Check sheet for the drawn part. Datum: minimum x, y, z corner. Units: mm. Round coordinates to 2 decimals unless told otherwise and drop trailing zeros. Write each loop counter-clockwise with the first axis right and the second up, starting at its lowest first coordinate (ties: lowest second). Pieces come first, ordered by that corner, then holes. Notation, with made-up numbers: M 15,79 L 64,79 A18 ccw 64,99 Z; hole C 57,-12.75 d10. An arc over 180 degrees is marked long. One line per item, written item: value. Start each with the question number.
Item 1: Section check B-B, the plane z = 43.5. Record the cut outline in (x, y).
Item 2: Gauge pin test, flat ends, axial feed: pin 1 (8 mm diameter, centred on y = 21.5, z = 21.5, fed in from +X) (1 decimal); pin 2 (1.5 mm diameter, centred on x = 97, y = 16, fed in from -Z) (1 decimal); pin 3 (4 mm diameter, centred on y = 16.5, z = 13.5, fed in from +X). Record the tip position at first contact, or that the pin passes through.
Item 3: Section check D-D, the plane x = 102. Record the cut outline in (y, z), then the cut area to 3 significant figures.
Item 4: Draft check along X on the marked faces 1, 2, 3 and 4. Enter one of: +X half, -X half, draft (parallel to the pull), parting line (faces both ways), or undercut.
Item 5: Section check A-A, the plane x = 61. Record the cut outline in (y, z), then the cut area to 3 significant figures.
Item 6: Thickness scan on probe 1 along Z at (x, y) = (54.5, 42.5) (1 decimal); probe 2 along X at (y, z) = (3, 37) (1 decimal); probe 3 along X at (y, z) = (21, 74.5) (1 decimal). Record the ranges inside material, lowest first. Write a range as from..to.
Item 7: Section check C-C, the plane y = 11. Record the cut outline in (x, z) (1 decimal), then the cut area to 3 significant figures.
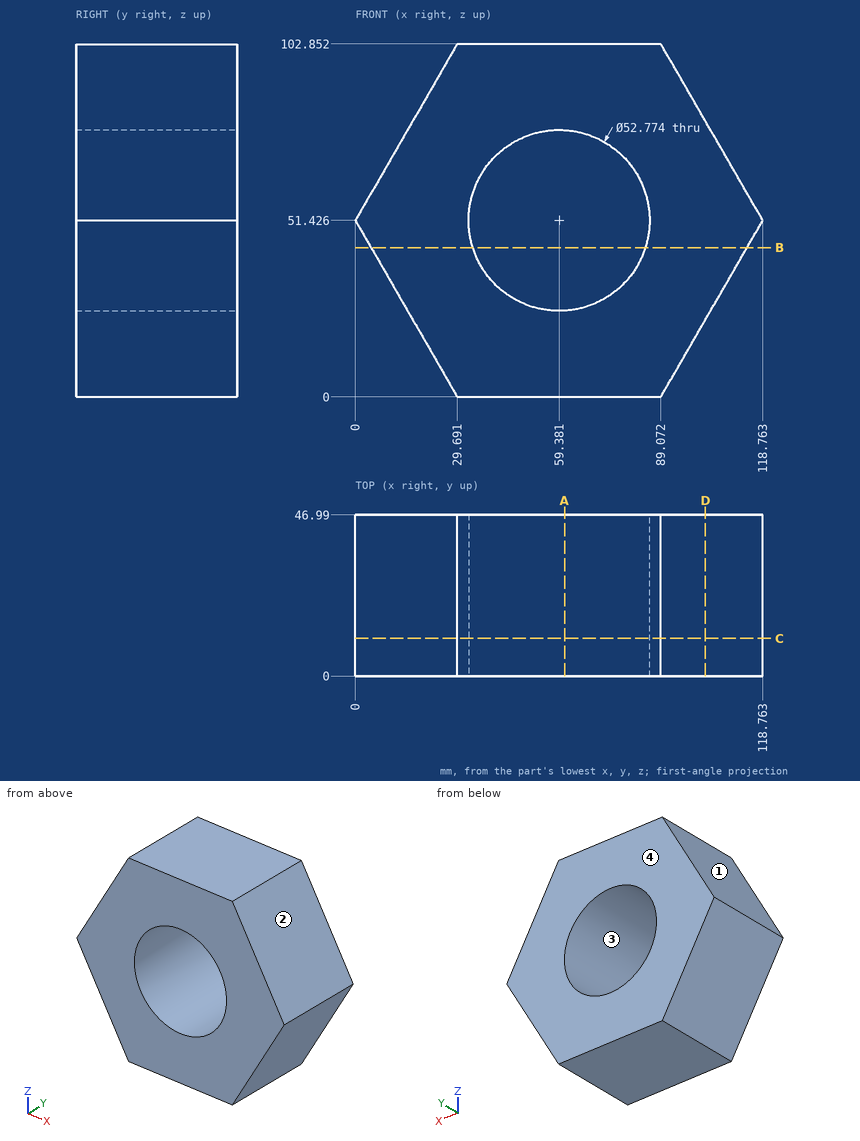
Response values:
1. outline: M 4.58,0 L 34.21,0 L 34.21,46.99 L 4.58,46.99 Z; M 84.55,0 L 114.19,0 L 114.19,46.99 L 84.55,46.99 Z
2. pin 1: stops at x = 103.8
2. pin 2: stops at z = 12.4
2. pin 3: stops at x = 98.02
3. outline: M 0,22.39 L 46.99,22.39 L 46.99,80.46 L 0,80.46 Z
3. area: 2,730 mm2
4. face 1: -X half
4. face 2: +X half
4. face 3: undercut
4. face 4: draft
5. outline: M 0,0 L 46.99,0 L 46.99,25.09 L 0,25.09 Z; M 0,77.76 L 46.99,77.76 L 46.99,102.85 L 0,102.85 Z
5. area: 2,360 mm2
6. probe 1: z = 0..25.5, 77.4..102.9
6. probe 2: x = 8.3..37.3, 81.5..110.4
6. probe 3: x = 13.3..46.6, 72.2..105.4
7. outline: M 0,51.4 L 29.7,0 L 89.1,0 L 118.8,51.4 L 89.1,102.9 L 29.7,102.9 Z; hole C 59.4,51.4 d52.8
7. area: 6,970 mm2
